```python
from build123d import *

# Parameters (mm, degrees)
F0_R     = 11.90625
F1_DEPTH = 25.4
F0_W     = 19.05
F0_H     = 15.875
F0_W_2   = 38.1
F2_DEPTH = 57.15


with BuildPart() as f1:
    # F0 (on Top) → F1 (new body)
    with BuildSketch(Plane.XY):
        Polygon((-57.15, -29.36875), (57.15, -29.36875), (57.15, 13.49375), (38.1, 13.49375), (0, 13.49375), (-38.1, 13.49375), (-57.15, 13.49375), align=None)
        with Locations((0, -7.14375)):
            Circle(F0_R, mode=Mode.SUBTRACT)
    extrude(amount=F1_DEPTH)

    # F0 (on Top) → F2 (join)
    with BuildSketch(Plane.XY):
        with Locations((-47.625, 21.43125)):
            Rectangle(F0_W, F0_H)
        with Locations((-19.05, 21.43125)):
            Rectangle(F0_W_2, F0_H)
        with Locations((19.05, 21.43125)):
            Rectangle(F0_W_2, F0_H)
        with Locations((47.625, 21.43125)):
            Rectangle(F0_W, F0_H)
    extrude(amount=F2_DEPTH)


solid = f1.part
```
For this review, take the finished solid that the model builds, in its own axes (mm). A direction names the side the tool comes from. Coordinates: 2 decimals unless noted, no trailing zeros. Loops run counter-clockwise (first coordinate to the right, second up) from the corner with the lowest first, then second, coordinate; pieces in that order, holes last. Notation, with made-up numbers: (23.25, 67.5) - (79.25, 67.5) arc R25 cw to (79.25, 102.5) - close; hole circle Ø8 at (31, -17.75). An arc over 180 degrees is marked (long way). Use one line per item in the form item = value. Start each with the question number.
1) Take a section at A-A (x = 0). State the section outline as (y, z) points, plus the area to 3 significant figures.
2) To check wall thickness, follow probe 1 along Y at (x, z) = (0, 12.75); probe 2 along Y at (x, z) = (18.5, 44); probe 3 along Z at (x, y) = (13, 12). State the ranges of each line that lie inside material, in increasing order. Write a range as from..to.
3) For faces 1 (the face through (1, 29.369, 28)), 2 (the face through (-14, -8, 25.4)), list the 3-axis set-ups (+Z, -Z, +X, -X, +Y, -Y) from which the entire face can be reached by the end or side of a thin tool; tool diameter is ignored.
4) Take a section at D-D (y = -5.5). State the section outline as (x, z) points.
5) Take a section at C-C (x = 49.5). State the section outline as (y, z) points, plus the area to 3 significant figures.
6) Take a section at B-B (y = -14.5). State the section outline as (x, z) points, plus the area to 3 significant figures.
7) For pin 1 (8 mm diameter, centred on y = -4, z = 30.5, fed in from -X); pin 2 (12 mm diameter, centred on x = 39.5, y = -23, fed in from +Z); pin 3 (5 mm diameter, centred on y = -19.5, z = 27.5, fed in from +X), all flat-tipped, find the tip position at first contact; note any pin that passes through.
8) Draft analysis for pull direction Y (two halves, no side actions). For faces 3 (the face through (-1, -29.369, 13)), 4 (the face through (-57.15, 6, 15)), 5 (the face through (-9.448, -14.389, 12.522)), state which applies: released by +Y, released by -Y, zero draft, split by the parting line, or undercut.
From the geometry:
q1.outline = (-29.37, 0) - (-19.05, 0) - (-19.05, 25.4) - (-29.37, 25.4) - close; (4.76, 0) - (29.37, 0) - (29.37, 57.15) - (13.49, 57.15) - (13.49, 25.4) - (4.76, 25.4) - close
q1.area = 1,390 mm2
q2.probe_1 = -29.37..-19.05, 4.76..29.37
q2.probe_2 = 13.49..29.37
q2.probe_3 = 0..25.4
q3.face_1 = +Z, -Z, +X, -X, +Y
q3.face_2 = +Z, +X, -X, -Y
q4.outline = (-57.15, 0) - (-11.79, 0) - (-11.79, 25.4) - (-57.15, 25.4) - close; (11.79, 0) - (57.15, 0) - (57.15, 25.4) - (11.79, 25.4) - close
q5.outline = (-29.37, 0) - (29.37, 0) - (29.37, 57.15) - (13.49, 57.15) - (13.49, 25.4) - (-29.37, 25.4) - close
q5.area = 2,000 mm2
q6.outline = (-57.15, 0) - (-9.36, 0) - (-9.36, 25.4) - (-57.15, 25.4) - close; (9.36, 0) - (57.15, 0) - (57.15, 25.4) - (9.36, 25.4) - close
q6.area = 2,430 mm2
q7.pin_1 = through
q7.pin_2 = 25.4
q7.pin_3 = 57.15
q8.face_3 = released by -Y
q8.face_4 = zero draft
q8.face_5 = undercut
